from build123d import *

# Parameters (mm, degrees)
SKETCH_1_W          = 64
SKETCH_1_H          = 76
SKETCH_1_R          = 2.25
SKETCH_1_R_2        = 1.7
EXTRUDE_1_DEPTH     = 2.5
EXTRUDE_START       = -20
SKETCH_2_W          = 5
SKETCH_2_H          = 61
EXTRUDE_2_DEPTH     = 2
EXTRUDE_2_2_DEPTH   = 2
SKETCH_3_W          = 2
SKETCH_3_H          = 11.5
EXTRUDE_3_DEPTH     = 20
SKETCH_4_W          = 6.5
SKETCH_4_H          = 2.5
EXTRUDE_4_DEPTH     = 20
SKETCH_5_R          = 10
CUT_EXTRUDE_1_DEPTH = 10


with BuildPart() as part:
    # Sketch 1 → Extrude 1 (new body)
    with BuildSketch(Plane(origin=(0, 0, 0), x_dir=(1, 0, 0), z_dir=(0, 1, 0))):
        Rectangle(SKETCH_1_W, SKETCH_1_H)
        with Locations(Location((-15.25, 15.25, 0), (0, 0, 270))):
            Circle(SKETCH_1_R, mode=Mode.SUBTRACT)
        with Locations(Location((-24, -33, 0), (0, 0, 270))):
            Circle(SKETCH_1_R_2, mode=Mode.SUBTRACT)
        with Locations(Location((24, -33, 0), (0, 0, 90))):
            Circle(SKETCH_1_R_2, mode=Mode.SUBTRACT)
        with Locations(Location((24, 33, 0), (0, 0, 270))):
            Circle(SKETCH_1_R_2, mode=Mode.SUBTRACT)
        with Locations(Location((-24, 33, 0), (0, 0, 90))):
            Circle(SKETCH_1_R_2, mode=Mode.SUBTRACT)
        with Locations(Location((15.25, 15.25, 0), (0, 0, 90))):
            Circle(SKETCH_1_R, mode=Mode.SUBTRACT)
        with Locations(Location((15.25, -15.25, 0), (0, 0, 270))):
            Circle(SKETCH_1_R, mode=Mode.SUBTRACT)
        with Locations(Location((-15.25, -15.25, 0), (0, 0, 90))):
            Circle(SKETCH_1_R, mode=Mode.SUBTRACT)
    extrude(amount=EXTRUDE_1_DEPTH)



with BuildPart() as body_2:
    # Sketch 2 → Extrude 2 (new body)
    with BuildSketch(Plane(origin=(0, 0, 0), x_dir=(1, 0, 0), z_dir=(0, 1, 0)).offset(EXTRUDE_START)):
        with Locations((14.5, 0)):
            Rectangle(SKETCH_2_W, SKETCH_2_H)
    extrude(amount=EXTRUDE_2_DEPTH)


with BuildPart() as body_3:
    # Sketch 2 → Extrude 2 2 (new body)
    with BuildSketch(Plane(origin=(0, 0, 0), x_dir=(1, 0, 0), z_dir=(0, 1, 0)).offset(EXTRUDE_START)):
        with Locations((-14.5, 0)):
            Rectangle(SKETCH_2_W, SKETCH_2_H)
    extrude(amount=EXTRUDE_2_2_DEPTH)


with BuildPart() as part_1:
    add(part.part)

    add(body_2.part)  # Extrude 3 merges body 2

    add(body_3.part)  # Extrude 3 merges body 3
    # Sketch 3 → Extrude 3 (add)
    with BuildSketch(Plane(origin=(0, 0, 0), x_dir=(1, 0, 0), z_dir=(0, 1, 0)).offset(EXTRUDE_START)):
        with Locations((17.5, -24.75)):
            Rectangle(SKETCH_3_W, SKETCH_3_H)
        with Locations((-17.5, -24.75)):
            Rectangle(SKETCH_3_W, SKETCH_3_H)
        Polygon((16.5, -1), (16.5, 11.5), (18.5, 11.5), (18.5, -1), (18.5, -11.5), (16.5, -11.5), align=None)
        with Locations((17.5, 24.75)):
            Rectangle(SKETCH_3_W, SKETCH_3_H)
        Polygon((-18.5, -1), (-18.5, 11.5), (-16.5, 11.5), (-16.5, -1), (-16.5, -11.5), (-18.5, -11.5), align=None)
        with Locations((-17.5, 24.75)):
            Rectangle(SKETCH_3_W, SKETCH_3_H)
    extrude(amount=EXTRUDE_3_DEPTH)

    # Sketch 4 → Extrude 4 (add)
    with BuildSketch(Plane(origin=(0, 0, 0), x_dir=(1, 0, 0), z_dir=(0, 1, 0)).offset(EXTRUDE_START)):
        with Locations((-15.25, -31.25)):
            Rectangle(SKETCH_4_W, SKETCH_4_H)
        with Locations((15.25, -31.25)):
            Rectangle(SKETCH_4_W, SKETCH_4_H)
    extrude(amount=EXTRUDE_4_DEPTH)

    # Sketch 5 → Cut-Extrude 1 (cut)
    with BuildSketch(Plane.XZ):
        with Locations(Location((0, 0, 0), (0, 0, 270))):
            Circle(SKETCH_5_R)
        Polygon((-22, 20), (-22, -20), (-32, -25.773502692), (-32, 25.773502692), align=None)
        Polygon((22, 20), (32, 25.773502692), (32, -25.773502692), (22, -20), align=None)
        Polygon((-17.5, 38), (17.5, 38), (9, 29.5), (9, 25.5), (-9, 25.5), (-9, 29.5), align=None)
        Polygon((-32, -25.875644347), (-25, -38), (-32, -38), align=None)
        Polygon((32, -25.875644347), (32, -38), (25, -38), align=None)
        Polygon((32, 25.875644347), (25, 38), (32, 38), align=None)
        Polygon((-32, 25.875644347), (-32, 38), (-25, 38), align=None)
        Polygon((17.5, -38), (9, -29.5), (9, -25.5), (-9, -25.5), (-9, -29.5), (-17.5, -38), align=None)
    extrude(amount=-CUT_EXTRUDE_1_DEPTH, mode=Mode.SUBTRACT)


solid = part_1.part
Can you work these out from the model? Positions are in its coordinate system, mm. A direction names the side the tool comes from. Give positions to 0.01 mm unless a question says otherwise; leave off trailing zeros. Write each loop counter-clockwise with the first axis right and the second up, starting at its lowest first coordinate (ties: lowest second). Pieces come first, ordered by that corner, then holes. Notation, with made-up numbers: M 76,-31 L 112,-31 A22 cw 112,-16 Z; hole C 88,8 d7. An arc over 180 degrees is marked long. Answer in a Markdown table with one row per item. Add a question column.
Item 1: On a 3-axis mill with a long thin cutter (end or side, diameter ignored), from which of +Z, -Z, +X, -X, +Y, -Y can I reach the whole of each face in a straight line? I mean faces 1 (the cylindrical face through (-13.254, 1.232, 14.212)), 2 (the flat face through (0, 1, -25.5)), 3 (the flat face through (-18.5, -10, 26)). Say none if no direction works.
Item 2: Please list where these lines run through material, in increasing order: L1, parallel to X at y = 1.7, z = -15.25; L2, parallel to Z at x = -17, y = -2; L3, parallel to X at y = -2.75, z = 0.5.
Item 3: Imagine slicing it at A-A, the plane z = 0. Write out the boundary of the cut face in (x, y).
Item 4: Imagine slicing it at D-D, the plane x = 0. Write out the boundary of the cut face in (y, z).
Item 5: For pin 1 Ø6 at (y, z) = (-4.5, -18.5) entering from +X; pin 2 Ø1.5 at (x, z) = (-15.5, 14.5) entering from +Y; pin 3 Ø1 at (x, y) = (17.5, -6) entering from +Z, each with a flat end and sliding along its axis, tell me the tip position at first contact or that it passes through.
Item 6: We'd pull the mould along X, two halves only. Please class faces 4 (the flat face through (-15, -20, 1)), 5 (the flat face through (-28.55, 1.23, -31.85)), 6 (the flat face through (22, 1, 0)), 7 (the flat face through (-14, -9, 30)): released by +X, released by -X, zero draft, split by the parting line, or undercut.
Item 7: Imagine slicing it at B-B, the plane y = -6. Write out the boundary of the cut face in (x, z), plus the area to 4 significant figures.
Item 8: Imagine slicing it at C-C, the plane z = 15.25. Write out the boundary of the cut face in (x, y).
Evaluation:
| question | item | result |
|---|---|---|
| 1 | face 1 | +Y |
| 1 | face 2 | -Z, +Y, -Y |
| 1 | face 3 | +Z, -Z, -X, -Y |
| 2 | L1 | x = -22 to -17.5, -13 to 13, 17.5 to 22 |
| 2 | L2 | z = -30.5 to -19, -11.5 to 11.5, 19 to 32.5 |
| 2 | L3 | x = -18.5 to -16.5, 16.5 to 18.5 |
| 3 | outline | M -22,0 L -18.5,0 L -18.5,-20 L -12,-20 L -12,-18 L -16.5,-18 L -16.5,0 L -10,0 L -10,2.5 L -22,2.5 Z; M 10,0 L 16.5,0 L 16.5,-18 L 12,-18 L 12,-20 L 18.5,-20 L 18.5,0 L 22,0 L 22,2.5 L 10,2.5 Z |
| 4 | outline | M 0,-25.5 L 2.5,-25.5 L 2.5,-10 L 0,-10 Z; M 0,10 L 2.5,10 L 2.5,25.5 L 0,25.5 Z |
| 5 | pin 1 | stops at x = 18.5 |
| 5 | pin 2 | stops at y = -18 |
| 5 | pin 3 | stops at z = 32.5 |
| 6 | face 4 | zero draft |
| 6 | face 5 | released by -X |
| 6 | face 6 | released by +X |
| 6 | face 7 | undercut |
| 7 | outline | M -18.5,-30.5 L -16.5,-30.5 L -16.5,-19 L -18.5,-19 Z; M -18.5,-11.5 L -16.5,-11.5 L -16.5,11.5 L -18.5,11.5 Z; M -18.5,19 L -16.5,19 L -16.5,30 L -12,30 L -12,32.5 L -18.5,32.5 Z; M 12,30 L 16.5,30 L 16.5,19 L 18.5,19 L 18.5,32.5 L 12,32.5 Z; M 16.5,-30.5 L 18.5,-30.5 L 18.5,-19 L 16.5,-19 Z; M 16.5,-11.5 L 18.5,-11.5 L 18.5,11.5 L 16.5,11.5 Z |
| 7 | area | 214.5 mm² |
| 8 | outline | M -22,0 L -17.5,0 L -17.5,2.5 L -22,2.5 Z; M -17,-20 L -12,-20 L -12,-18 L -17,-18 Z; M -13,0 L 13,0 L 13,2.5 L -13,2.5 Z; M 12,-20 L 17,-20 L 17,-18 L 12,-18 Z; M 17.5,0 L 22,0 L 22,2.5 L 17.5,2.5 Z |
